from build123d import *

# Parameters (mm, degrees)
SKETCH1_R      = 1.35
SKETCH1_R_2    = 1.25
EXTRUDE1_DEPTH = 3.1


with BuildPart() as part:
    # Sketch1 → Extrude1 (new body)
    with BuildSketch(Plane.XY):
        with BuildLine():
            Line((-24.241802054, 13.266728144), (-19.191802054, 13.266728144))
            Line((-19.191802054, 13.266728144), (12.808197946, 13.266728144))
            Line((12.808197946, 13.266728144), (17.858197946, 13.266728144))
            ThreePointArc((17.858197946, 13.266728144), (21.733197946, 9.391728144), (17.858197946, 5.516728144))
            Line((17.858197946, 5.516728144), (12.808197946, 5.516728144))
            Line((12.808197946, 5.516728144), (12.808197946, -9.483271856))
            Line((12.808197946, -9.483271856), (17.858197946, -9.483271856))
            ThreePointArc((17.858197946, -9.483271856), (21.733197946, -13.358271856), (17.858197946, -17.233271856))
            Line((17.858197946, -17.233271856), (12.808197946, -17.233271856))
            Line((12.808197946, -17.233271856), (-19.191802054, -17.233271856))
            Line((-19.191802054, -17.233271856), (-24.241802054, -17.233271856))
            ThreePointArc((-24.241802054, -17.233271856), (-28.116802054, -13.358271856), (-24.241802054, -9.483271856))
            Line((-24.241802054, -9.483271856), (-19.191802054, -9.483271856))
            Line((-19.191802054, -9.483271856), (-19.191802054, 5.516728144))
            Line((-19.191802054, 5.516728144), (-24.241802054, 5.516728144))
            ThreePointArc((-24.241802054, 5.516728144), (-28.116802054, 9.391728144), (-24.241802054, 13.266728144))
        make_face()
        with Locations(Location((-14.806030935, 9.630953317, 0), (0, 0, 180))):
            Circle(SKETCH1_R, mode=Mode.SUBTRACT)
        with Locations(Location((8.422426827, -13.597504445, 0), (0, 0, 180))):
            Circle(SKETCH1_R, mode=Mode.SUBTRACT)
        with Locations(Location((-14.806030935, -13.597504445, 0), (0, 0, 180))):
            Circle(SKETCH1_R, mode=Mode.SUBTRACT)
        with Locations(Location((8.422426827, 9.630953317, 0), (0, 0, 180))):
            Circle(SKETCH1_R, mode=Mode.SUBTRACT)
        with Locations(Location((-24.241802054, 9.414269496, 0), (0, 0, 180))):
            Circle(SKETCH1_R_2, mode=Mode.SUBTRACT)
        with Locations(Location((-24.241802054, -13.380813208, 0), (0, 0, 180))):
            Circle(SKETCH1_R_2, mode=Mode.SUBTRACT)
        with Locations(Location((17.858197946, -13.380813208, 0), (0, 0, 180))):
            Circle(SKETCH1_R_2, mode=Mode.SUBTRACT)
        with Locations(Location((17.858197946, 9.414269496, 0), (0, 0, 180))):
            Circle(SKETCH1_R_2, mode=Mode.SUBTRACT)
        with BuildLine():
            Line((-13.191802054, 4.016724436), (-13.191802054, -7.983275564))
            ThreePointArc((-13.191802054, -7.983275564), (-12.020229179, -10.811702689), (-9.191802054, -11.983275564))
            Line((-9.191802054, -11.983275564), (2.808197946, -11.983275564))
            ThreePointArc((2.808197946, -11.983275564), (5.636625071, -10.811702689), (6.808197946, -7.983275564))
            Line((6.808197946, -7.983275564), (6.808197946, 4.016724436))
            ThreePointArc((6.808197946, 4.016724436), (5.636625071, 6.84515156), (2.808197946, 8.016724436))
            Line((2.808197946, 8.016724436), (-9.191802054, 8.016724436))
            ThreePointArc((-9.191802054, 8.016724436), (-12.020229179, 6.84515156), (-13.191802054, 4.016724436))
        make_face(mode=Mode.SUBTRACT)
    extrude(amount=EXTRUDE1_DEPTH)


solid = part.part
Design review of the part built by this model. Coordinates are the model's own, in mm. A direction names the side the tool comes from. Coordinates: 2 decimals unless noted, no trailing zeros. Write each loop counter-clockwise with the first axis right and the second up, starting at its lowest first coordinate (ties: lowest second). Pieces come first, ordered by that corner, then holes. Notation, with made-up numbers: (23.5, 67.5) - (37.5, 67.5) arc R20 ccw to (37.5, 79.5) - close; hole circle Ø4 at (34, 73). An arc over 180 degrees is marked (long way). One line per item, written item: value.
1) Mouldability with a two-part tool opening along Y and no side actions: class faces 4 (the face through (-3, 13.267, 2)), 5 (the face through (15, -9.483, 2)), 6 (the face through (-2.8, 8.4, 3.1)), 7 (the face through (-19.192, -2, 2)) as +Y half, -Y half, draft (parallel to the pull), parting line (faces both ways), or undercut.
Answer sheet:
face 4: +Y half
face 5: undercut
face 6: draft
face 7: undercut
2) For faces 1 (the face through (-3, 8.017, 2)), 2 (the face through (-22, 5.517, 2)), 3 (the face through (15, 5.517, 2)), list the 3-axis set-ups (+Z, -Z, +X, -X, +Y, -Y) from which the entire face can be reached by the end or side of a thin tool; tool diameter is ignored.
Answer sheet:
face 1: +Z, -Z
face 2: +Z, -Z, -X
face 3: +Z, -Z, +X
3) Add section D-D (z = 2.5). Give the number of separate pieces and of enclosed holes in the cut face, plus the area to 3 significant figures.
Answer sheet:
separate pieces: 1
enclosed holes: 9
area: 798 mm2
4) Insertion check: pin 1 (1 mm diameter, centred on y = 6.5, z = 1.5, fed in from -X); pin 2 (0.9 mm diameter, centred on y = -5, z = 2.5, fed in from -X). Each pin has a flat end and moves straight along its axis. Give the tip position at first contact, or say it passes through.
Answer sheet:
pin 1: stops at x = -27.29
pin 2: stops at x = -19.19
5) Add section C-C (x = -15.5). State the section outline as (y, z) points.
Answer sheet:
outline: (-17.23, 0) - (-14.76, 0) - (-14.76, 3.1) - (-17.23, 3.1) - close; (-12.44, 0) - (8.47, 0) - (8.47, 3.1) - (-12.44, 3.1) - close; (10.79, 0) - (13.27, 0) - (13.27, 3.1) - (10.79, 3.1) - close
6) Add section B-B (y = -5). State the section outline as (x, z) points.
Answer sheet:
outline: (-19.19, 0) - (-13.19, 0) - (-13.19, 3.1) - (-19.19, 3.1) - close; (6.81, 0) - (12.81, 0) - (12.81, 3.1) - (6.81, 3.1) - close
7) To check wall thickness, follow probe 1 along X at (y, z) = (-6, 2.9); probe 2 along Y at (x, z) = (3, 1.2); probe 3 along Y at (x, z) = (13, 2.85). State the ranges of each line that lie inside material, in increasing order.
Answer sheet:
probe 1: x = -19.19 to -13.19, 6.81 to 12.81
probe 2: y = -17.23 to -11.98, 8.01 to 13.27
probe 3: y = -17.23 to -9.48, 5.52 to 13.27
8) Add section A-A (x = 16). State the section outline as (y, z) points.
Answer sheet:
outline: (-17.23, 0) - (-9.48, 0) - (-9.48, 3.1) - (-17.23, 3.1) - close; (5.52, 0) - (13.27, 0) - (13.27, 3.1) - (5.52, 3.1) - close
